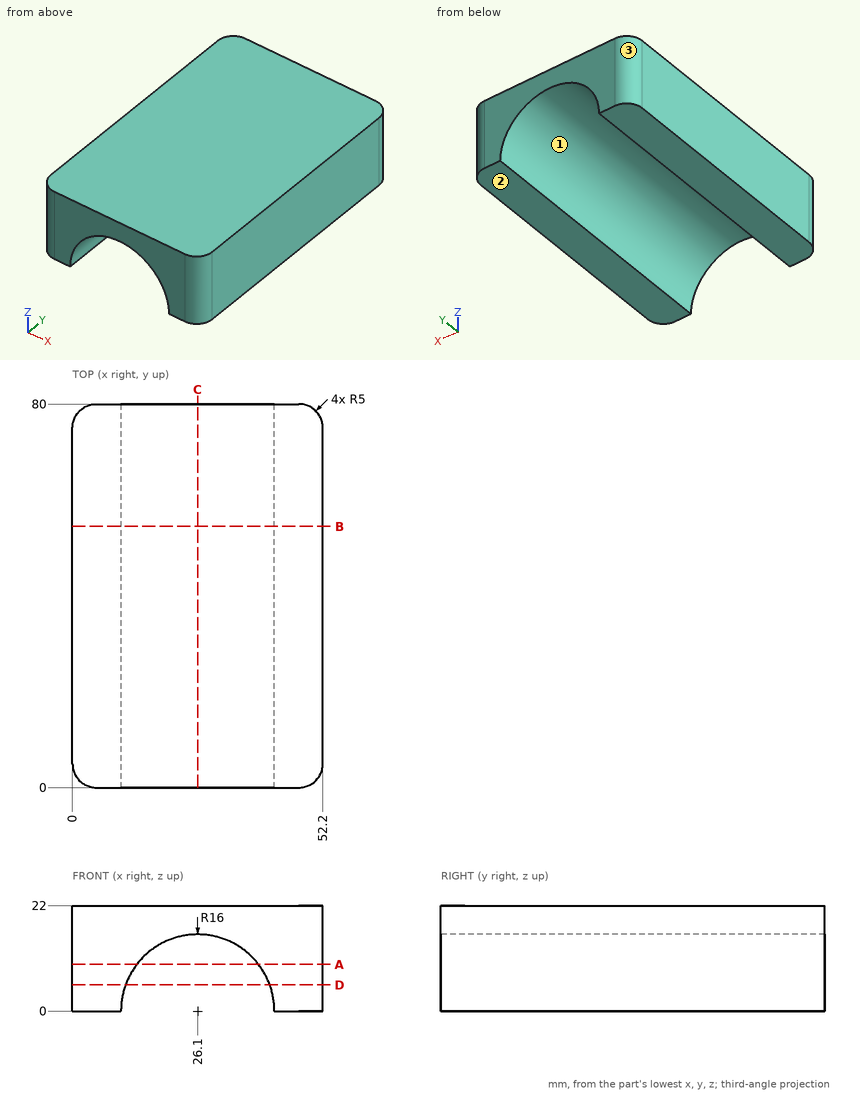
Verification items for this drawing (mm, ordinates from the low corner). Coordinates: 2 decimals unless noted, no trailing zeros. Loops run counter-clockwise (first coordinate to the right, second up) from the corner with the lowest first, then second, coordinate; pieces in that order, holes last. Notation, with made-up numbers: (-20.5, -27) - (-4.5, -27) arc R17 cw to (-4.5, -9) - close; hole circle Ø8 at (26, 40.5). An arc over 180 degrees is marked (long way). Use one line per item in the form item = value. Start each with the question number.
Item 1: Section check A-A, the plane z = 9.75. Enter the section's corners in (x, y).
Item 2: Gauge pin test, flat ends, axial feed: pin 1 (2 mm diameter, centred on x = 8.5, z = 4, fed in from -Y); pin 2 (5 mm diameter, centred on x = 32, y = 33.5, fed in from -Z); pin 3 (1 mm diameter, centred on x = 28, y = 56.5, fed in from -Z). Record the tip position at first contact, or that the pin passes through.
Item 3: Section check D-D, the plane z = 5.5. Enter the section's corners in (x, y), and give its area (3 significant figures).
Item 4: Section check B-B, the plane y = 54.5. Enter the section's corners in (x, z), and give its area (3 significant figures).
Item 5: Mould release check, pull along X, two halves, no side actions. Record for the marked faces 1, 2 and 3: +X half, -X half, draft (parallel to the pull), parting line (faces both ways), or undercut.
Item 6: Section check C-C, the plane x = 26.1. Enter the section's corners in (y, z), and give its area (3 significant figures).
Item 7: Thickness scan on probe 1 along X at (y, z) = (50.5, 8.25); probe 2 along X at (y, z) = (55, 10); probe 3 along Z at (x, y) = (33.5, 40.5). Record the ranges inside material, lowest first.
Computed:
q1.outline = (0, 5) arc R5 ccw to (5, 0) - (13.41, 0) - (13.41, 80) - (5, 80) arc R5 ccw to (0, 75) - close; (38.79, 0) - (47.2, 0) arc R5 ccw to (52.2, 5) - (52.2, 75) arc R5 ccw to (47.2, 80) - (38.79, 80) - close
q2.pin_1 = 0
q2.pin_2 = 13.62
q2.pin_3 = 15.82
q3.outline = (0, 5) arc R5 ccw to (5, 0) - (11.08, 0) - (11.08, 80) - (5, 80) arc R5 ccw to (0, 75) - close; (41.12, 0) - (47.2, 0) arc R5 ccw to (52.2, 5) - (52.2, 75) arc R5 ccw to (47.2, 80) - (41.12, 80) - close
q3.area = 1,750 mm2
q4.outline = (0, 0) - (10.1, 0) arc R16 cw to (42.1, 0) - (52.2, 0) - (52.2, 22) - (0, 22) - close
q4.area = 746 mm2
q5.face_1 = undercut
q5.face_2 = draft
q5.face_3 = -X half
q6.outline = (0, 16) - (80, 16) - (80, 22) - (0, 22) - close
q6.area = 480 mm2
q7.probe_1 = 0 to 12.39, 39.81 to 52.2
q7.probe_2 = 0 to 13.61, 38.59 to 52.2
q7.probe_3 = 14.19 to 22
